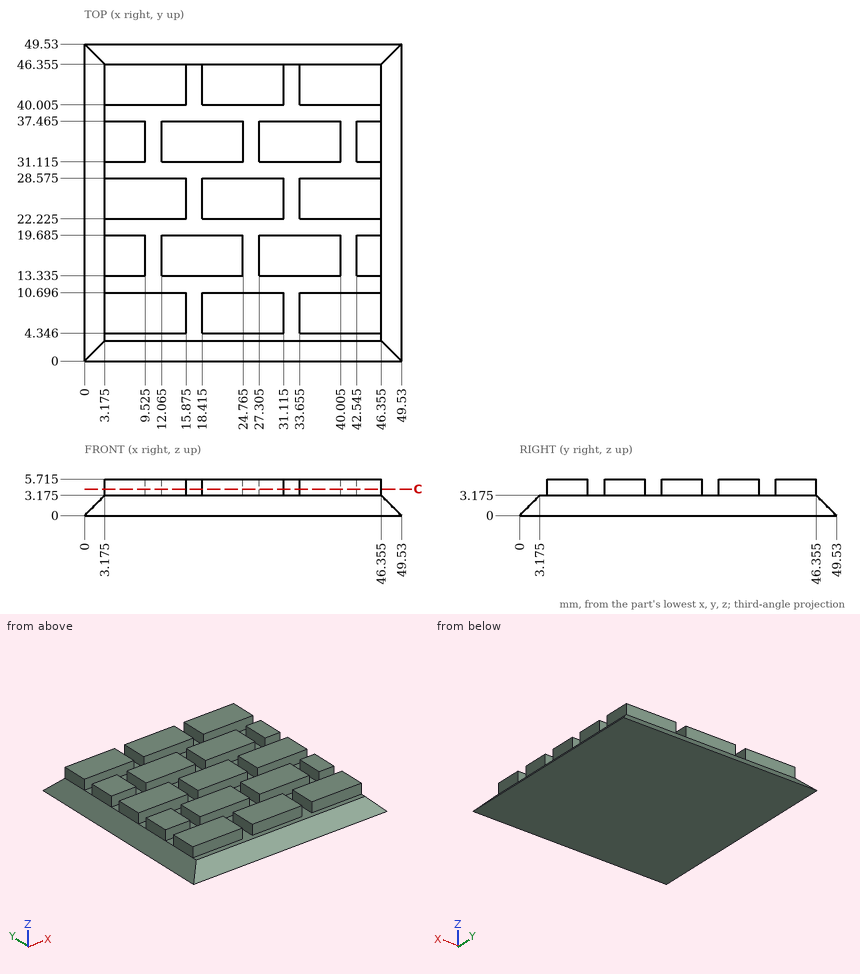
Geometry check sheet. Reference: drawing and pictorial views, mm from the part's lowest x, y, z. Give positions to 0.01 mm unless a question says otherwise; leave off trailing zeros. Answer in a Markdown table with one row per item. Add a question column.
Item 1: Gauge pin test, flat ends, axial feed: pin 1 (0.8 mm diameter, centred on y = 6.5, z = 5, fed in from -X) (3 decimals); pin 2 (3 mm diameter, centred on y = 25.5, z = 4, fed in from +X); pin 3 (0.8 mm diameter, centred on y = 15, z = 4.5, fed in from +X) (3 decimals). Record the tip position at first contact, or that the pin passes through.
Item 2: Section check C-C, the plane z = 4.15. State how many separate pieces and enclosed holes the cut face has, and give its area (3 significant figures).
Item 3: Scan lines: probe 1 along Y at (x, z) = (4.5, 4.1) (1 decimal); probe 2 along X at (y, z) = (16.5, 3.8) (1 decimal); probe 3 along X at (y, z) = (5, 4.6) (1 decimal). Record each from-to range of solid material in increasing order. Write a range as from..to.
Filled sheet:
| question | item | result |
|---|---|---|
| 1 | pin 1 | stops at x = 3.175 |
| 1 | pin 2 | stops at x = 47.03 |
| 1 | pin 3 | stops at x = 46.355 |
| 2 | separate pieces | 17 |
| 2 | enclosed holes | 0 |
| 2 | area | 1,180 mm^2 |
| 3 | probe 1 | y = 4.3..10.7, 13.3..19.7, 22.2..28.6, 31.1..37.5, 40..46.4 |
| 3 | probe 2 | x = 3.2..9.5, 12.1..24.8, 27.3..40, 42.5..46.4 |
| 3 | probe 3 | x = 3.2..15.9, 18.4..31.1, 33.7..46.4 |
